Design review of the part shown in the three views and the two pictorial views. Dimensions are in mm from the part's minimum x, y and z. A direction names the side the tool comes from. Give positions to 0.01 mm unless a question says otherwise; leave off trailing zeros. Order: outer loops, then holes, each group sorted by start corner. A loop starts at its lowest first (then second) coordinate and runs counter-clockwise, first axis right, second up. Notation, with made-up numbers: (2.5, -3.75) -> (10.5, -3.75) arc R14 cw to (10.5, 6.25) -> close; hole circle Ø2 at (28, -7.75). An arc over 180 degrees is marked (long way). Use one line per item in the form item = value.
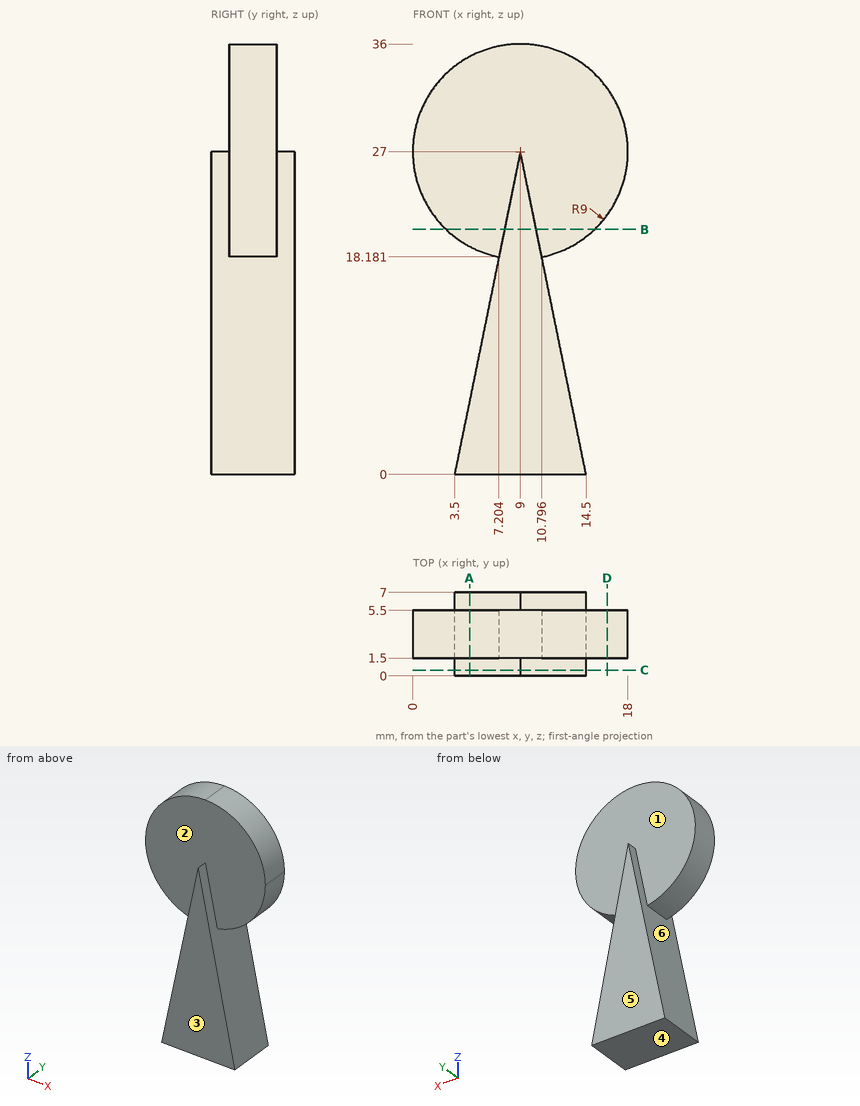
1. For pin 1 Ø5.5 at (x, z) = (9.5, 31) entering from +Y, flat-tipped, find the tip position at first contact; note if it passes through.
Values:
pin_1 = 5.5
2. Add section B-B on z = 20.5. Give the boundary of the cut face in (x, y) (1 decimal).
Values:
outline = (2.8, 1.5) -> (7.7, 1.5) -> (7.7, 0) -> (10.3, 0) -> (10.3, 1.5) -> (15.2, 1.5) -> (15.2, 5.5) -> (10.3, 5.5) -> (10.3, 7) -> (7.7, 7) -> (7.7, 5.5) -> (2.8, 5.5) -> close
3. Add section A-A on x = 4.75. Give the boundary of the cut face in (y, z), then the cut area to 3 significant figures.
Values:
outline = (0, 0) -> (7, 0) -> (7, 6.14) -> (0, 6.14) -> close; (1.5, 19.07) -> (5.5, 19.07) -> (5.5, 34.93) -> (1.5, 34.93) -> close
area = 106 mm^2
4. Add section C-C on y = 0.5. Give the boundary of the cut face in (x, z).
Values:
outline = (3.5, 0) -> (14.5, 0) -> (9, 27) -> close
5. Add section D-D on x = 16.25. Give the boundary of the cut face in (y, z).
Values:
outline = (1.5, 21.67) -> (5.5, 21.67) -> (5.5, 32.33) -> (1.5, 32.33) -> close
6. The part is to be moulded in two halves that separate along Z. For the marked faces 4, 5 and 6, say which applies: +Z half, -Z half, draft (parallel to the pull), parting line (faces both ways), or undercut.
Values:
face_4 = -Z half
face_5 = draft
face_6 = undercut
7. Tool access review of the marked faces 1, 2 and 3: name each direction out of +Z, -Z, +X, -X, +Y, -Y from which nothing blocks a thin tool from reaching the whole face with its end or side.
Values:
face_1 = +Z, +Y
face_2 = +Z, -Y
face_3 = +Z, -Z, +X, -X, -Y
8. For L1, parallel to Y at x = 10.25, z = 23.5; L2, parallel to Z at x = 8.75, y = 5.25; L3, parallel to X at y = 1, z = 21, list the stretches that pass through material, from the lowest coordinate up.
Values:
L1 = 1.5 to 5.5
L2 = 0 to 36
L3 = 7.78 to 10.22
